Could you check a few things on this drawing? It's one solid part, dimensions in mm from its lowest x, y, z. Give positions to 0.01 mm unless a question says otherwise; leave off trailing zeros. Write each loop counter-clockwise with the first axis right and the second up, starting at its lowest first coordinate (ties: lowest second). Pieces come first, ordered by that corner, then holes.
1. Suppose I cut it at B-B (x = 36.59). Please give me the cut outline in (y, z).
2. Suppose I cut it at C-C (y = 0.95). Please give me the cut outline in (x, z).
3. I'm going to push a flat-ended pin straight in: pin 1 (3 mm diameter, centred on x = 36.59, z = 33, fed in from +Y). Where does the tip first touch, or does it pass through?
4. Suppose I cut it at A-A (z = 3). Please give me the cut outline in (x, y).
5. Suppose I cut it at D-D (z = 11.5). Please give me the cut outline in (x, y).
6. If I drill on probe 1 along Z at (x, y) = (9.5, 1); probe 2 along Z at (x, y) = (6.59, 0.75); probe 3 along X at (y, z) = (0.6, 33), over which ranges is the centre line in solid material (lowest first)?
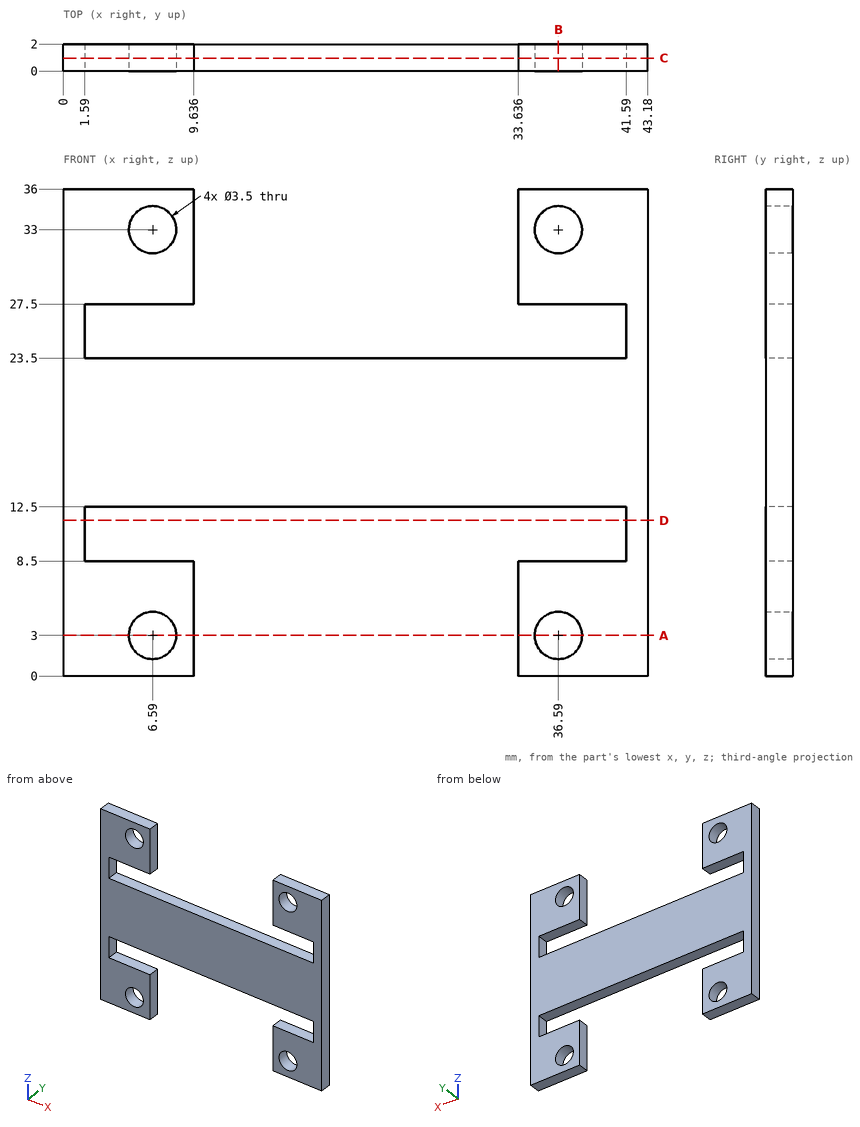
Checks:
1. outline: (0, 0) - (2, 0) - (2, 1.25) - (0, 1.25) - close; (0, 4.75) - (2, 4.75) - (2, 8.5) - (0, 8.5) - close; (0, 12.5) - (2, 12.5) - (2, 23.5) - (0, 23.5) - close; (0, 27.5) - (2, 27.5) - (2, 31.25) - (0, 31.25) - close; (0, 34.75) - (2, 34.75) - (2, 36) - (0, 36) - close
2. outline: (0, 0) - (9.64, 0) - (9.64, 8.5) - (1.59, 8.5) - (1.59, 12.5) - (41.59, 12.5) - (41.59, 8.5) - (33.64, 8.5) - (33.64, 0) - (43.18, 0) - (43.18, 36) - (33.64, 36) - (33.64, 27.5) - (41.59, 27.5) - (41.59, 23.5) - (1.59, 23.5) - (1.59, 27.5) - (9.64, 27.5) - (9.64, 36) - (0, 36) - close; hole circle Ø3.5 at (6.59, 3); hole circle Ø3.5 at (6.59, 33); hole circle Ø3.5 at (36.59, 3); hole circle Ø3.5 at (36.59, 33)
3. pin 1: passes through
4. outline: (0, 0) - (4.84, 0) - (4.84, 2) - (0, 2) - close; (8.34, 0) - (9.64, 0) - (9.64, 2) - (8.34, 2) - close; (33.64, 0) - (34.84, 0) - (34.84, 2) - (33.64, 2) - close; (38.34, 0) - (43.18, 0) - (43.18, 2) - (38.34, 2) - close
5. outline: (0, 0) - (1.59, 0) - (1.59, 2) - (0, 2) - close; (41.59, 0) - (43.18, 0) - (43.18, 2) - (41.59, 2) - close
6. probe 1: z = 0 to 8.5, 12.5 to 23.5, 27.5 to 36
6. probe 2: z = 0 to 1.25, 4.75 to 8.5, 12.5 to 23.5, 27.5 to 31.25, 34.75 to 36
6. probe 3: x = 0 to 4.84, 8.34 to 9.64, 33.64 to 34.84, 38.34 to 43.18
